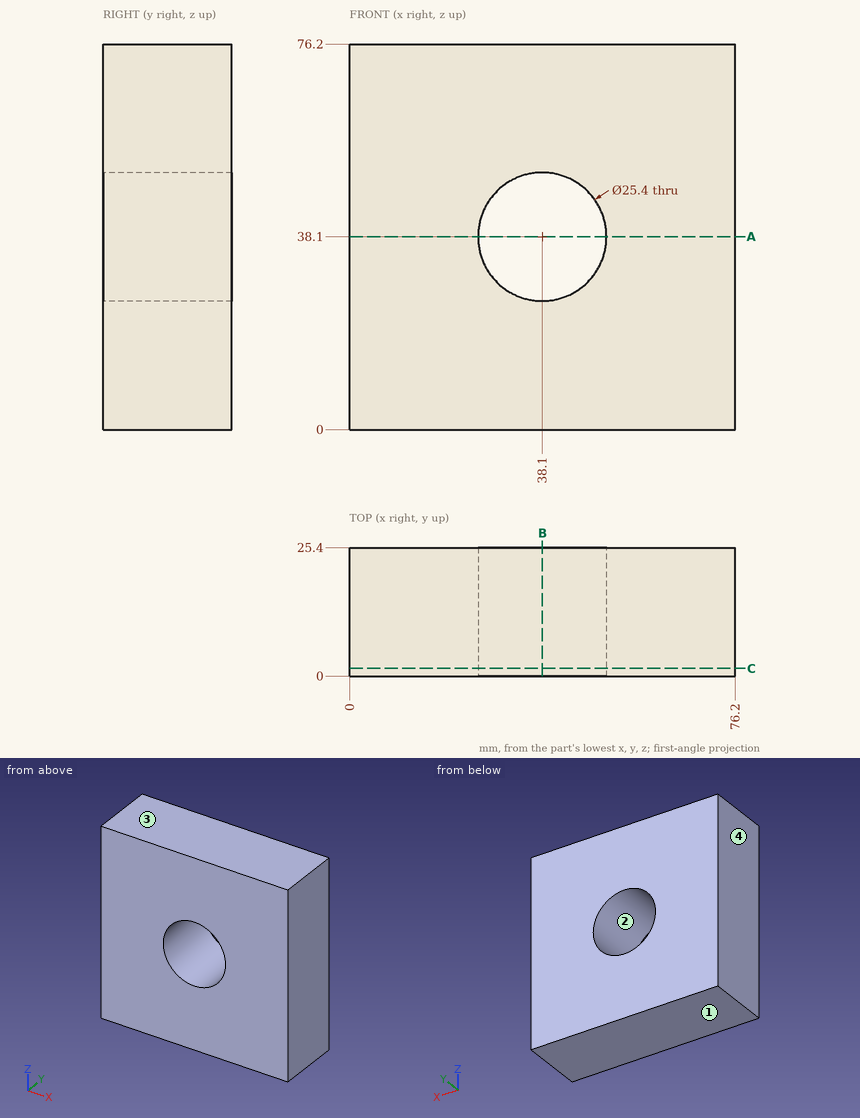
The drawing under review shows one solid part. Ordinate dimensions are in mm from its lowest x, y, z. Give positions to 0.01 mm unless a question says otherwise; leave off trailing zeros. Order: outer loops, then holes, each group sorted by start corner. A loop starts at its lowest first (then second) coordinate and runs counter-clockwise, first axis right, second up. Notation, with made-up numbers: M 75,48 L 130,48 A24 cw 130,65 Z; hole C 36.5,-34.5 d1. An arc over 180 degrees is marked long. Answer in a Markdown table with one row per item. Add a question column.
1. To check wall thickness, follow line 1 along Z through (x, y) = (38.1, 20); line 2 along X through (y, z) = (20.5, 27); line 3 along X through (y, z) = (7.5, 30). State the ranges of each line that lie inside material, in increasing order.
2. Add section B-B on x = 38.1. State the section outline as (y, z) points.
3. Add section A-A on z = 38.1. State the section outline as (x, y) points, plus the area to 3 significant figures.
4. Mouldability with a two-part tool opening along Z and no side actions: class the marked faces 1, 2, 3 and 4 as released by +Z, released by -Z, zero draft, split by the parting line, or undercut.
5. Add section C-C on y = 1.5. State the section outline as (x, z) points.
The answers:
| question | item | result |
|---|---|---|
| 1 | line 1 | 0 to 25.4, 50.8 to 76.2 |
| 1 | line 2 | 0 to 31.93, 44.27 to 76.2 |
| 1 | line 3 | 0 to 28.32, 47.88 to 76.2 |
| 2 | outline | M 0,0 L 25.4,0 L 25.4,25.4 L 0,25.4 Z; M 0,50.8 L 25.4,50.8 L 25.4,76.2 L 0,76.2 Z |
| 3 | outline | M 0,0 L 25.4,0 L 25.4,25.4 L 0,25.4 Z; M 50.8,0 L 76.2,0 L 76.2,25.4 L 50.8,25.4 Z |
| 3 | area | 1,290 mm2 |
| 4 | face 1 | released by -Z |
| 4 | face 2 | undercut |
| 4 | face 3 | released by +Z |
| 4 | face 4 | zero draft |
| 5 | outline | M 0,0 L 76.2,0 L 76.2,76.2 L 0,76.2 Z; hole C 38.1,38.1 d25.4 |
